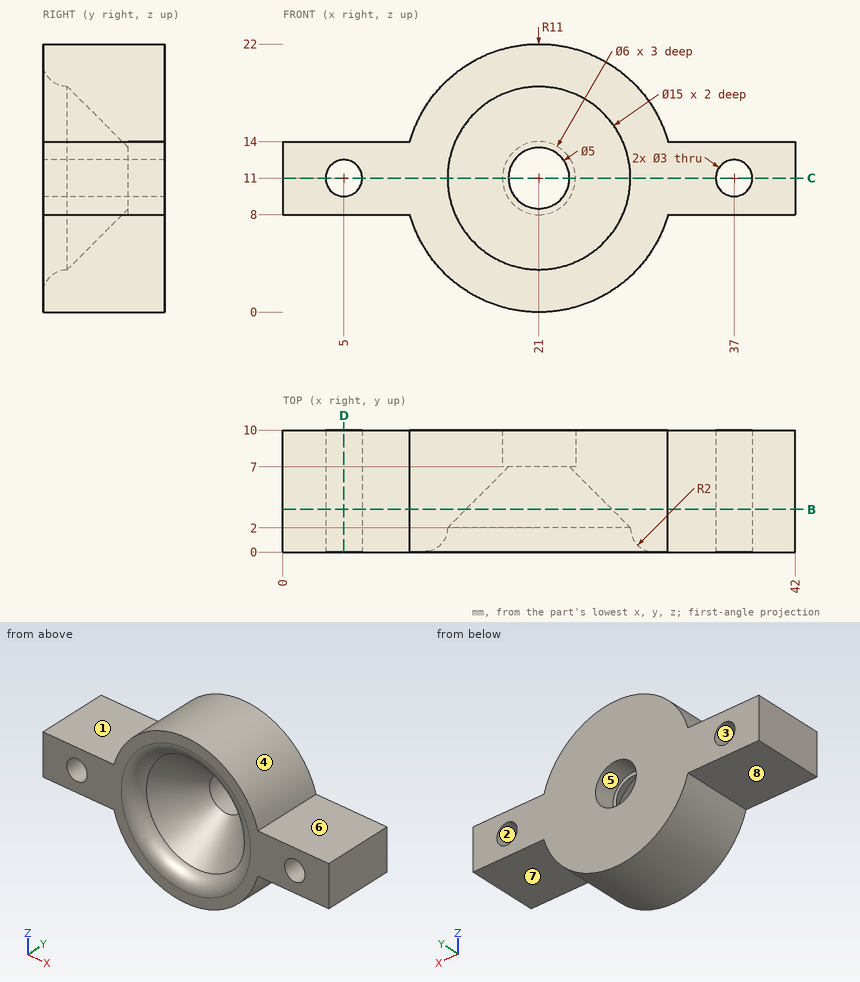
Check sheet for the drawn part. Datum: minimum x, y, z corner. Units: mm. A direction names the side the tool comes from. Coordinates: 2 decimals unless noted, no trailing zeros. Loops run counter-clockwise (first coordinate to the right, second up) from the corner with the lowest first, then second, coordinate; pieces in that order, holes last. Notation, with made-up numbers: (-5.75, 78.5) -> (13.25, 78.5) arc R21 cw to (13.25, 107.5) -> close; hole circle Ø8 at (26.5, 30). An arc over 180 degrees is marked (long way). Answer in a Markdown table with one row per item.
1. Sectioned sample at D-D, the plane x = 5. Record the boundary of the cut face in (y, z), then the cut area to 3 significant figures.
Check values:
| item | result |
|---|---|
| outline | (0, 8) -> (10, 8) -> (10, 9.5) -> (0, 9.5) -> close; (0, 12.5) -> (10, 12.5) -> (10, 14) -> (0, 14) -> close |
| area | 30.0 mm2 |
2. Release check for a two-part mould opening along X. For the marked faces 1, 2, 3 and 4 record: released by +X, released by -X, zero draft, split by the parting line, or undercut.
Check values:
| item | result |
|---|---|
| face 1 | zero draft |
| face 2 | undercut |
| face 3 | undercut |
| face 4 | split by the parting line |
3. Sectioned sample at C-C, the plane z = 11. Give the number of separate pieces and of enclosed holes in the cut face, then the cut area to 3 significant figures.
Check values:
| item | result |
|---|---|
| separate pieces | 4 |
| enclosed holes | 0 |
| area | 260 mm2 |
4. Material ranges on line 1 along X through (y, z) = (2, 11); line 2 along X through (y, z) = (7.75, 11); line 3 along Z through (x, y) = (24, 3.75) (1 decimal), recorded low to high. Write a range as [from, to].
Check values:
| item | result |
|---|---|
| line 1 | x = [0, 3.5], [6.5, 13.5], [28.5, 35.5], [38.5, 42] |
| line 2 | x = [0, 3.5], [6.5, 18], [24, 35.5], [38.5, 42] |
| line 3 | z = [0.4, 6.1], [15.9, 21.6] |
5. Sectioned sample at B-B, the plane y = 3.5. Record the boundary of the cut face in (x, z).
Check values:
| item | result |
|---|---|
| outline | (0, 8) -> (10.42, 8) arc R11 ccw to (31.58, 8) -> (42, 8) -> (42, 14) -> (31.58, 14) arc R11 ccw to (10.42, 14) -> (0, 14) -> close; hole circle Ø3 at (5, 11); hole circle Ø12 at (21, 11); hole circle Ø3 at (37, 11) |
6. Access from +Z, -Z, +X, -X, +Y, -Y to the whole of each face (thin tool, end or side, straight path). Record for the marked faces 5, 6, 7 and 8.
Check values:
| item | result |
|---|---|
| face 5 | +Y |
| face 6 | +Z, +X, +Y, -Y |
| face 7 | -Z, +X, +Y, -Y |
| face 8 | -Z, -X, +Y, -Y |
7. Go/stop test with flat-tipped pins: pin 1 (3 mm diameter, centred on x = 13.5, z = 8, fed in from -Y); pin 2 (3 mm diameter, centred on x = 39.5, y = 5, fed in from +Z); pin 3 (1.8 mm diameter, centred on x = 20.5, z = 11, fed in from +Y); pin 4 (3 mm diameter, centred on x = 35, y = 3, fed in from -Z). Record where each tip stops, or that it passes through.
Check values:
| item | result |
|---|---|
| pin 1 | stops at y = 0 |
| pin 2 | stops at z = 14 |
| pin 3 | passes through |
| pin 4 | stops at z = 8 |
